Could you check a few things on this drawing? It's one solid part, dimensions in mm from its lowest x, y, z. Round coordinates to 2 decimals unless told otherwise and drop trailing zeros. Write each loop counter-clockwise with the first axis right and the second up, starting at its lowest first coordinate (ties: lowest second). Pieces come first, ordered by that corner, then holes. Notation, with made-up numbers: (23.5, 60) - (72.5, 60) arc R37 cw to (72.5, 96) - close; hole circle Ø3 at (-10.5, 49). An arc over 180 degrees is marked (long way). Use one line per item in the form item = value. Start each with the question number.
1. I want a section at A-A, the plane z = 3.5. State how many separate pieces and enclosed holes the cut face has, plus the area to 3 significant figures.
2. Will these pins go through, and if not, where does the flat tip stop? pin 1 (2.5 mm diameter, centred on y = 167, z = 2, fed in from -X); pin 2 (1 mm diameter, centred on x = 187.5, z = 4, fed in from +Y); pin 3 (1.5 mm diameter, centred on x = 130.5, z = 2.5, fed in from -Y).
3. I want a section at B-B, the plane x = 91. List the corners of the cut face in (y, z) for me.
4. I want a section at D-D, the plane x = 44. List the corners of the cut face in (y, z) for me.
5. If I drill on line 1 along Y through (x, z) = (92, 3.85); line 2 along X through (y, z) = (69, 3.7); line 3 along Y through (x, z) = (132.5, 2.9), over which ranges is the centre line in solid material (lowest first)?
6. I want a section at C-C, the plane y = 148. List the corners of the cut face in (x, z) for me, plus the area to 3 significant figures.
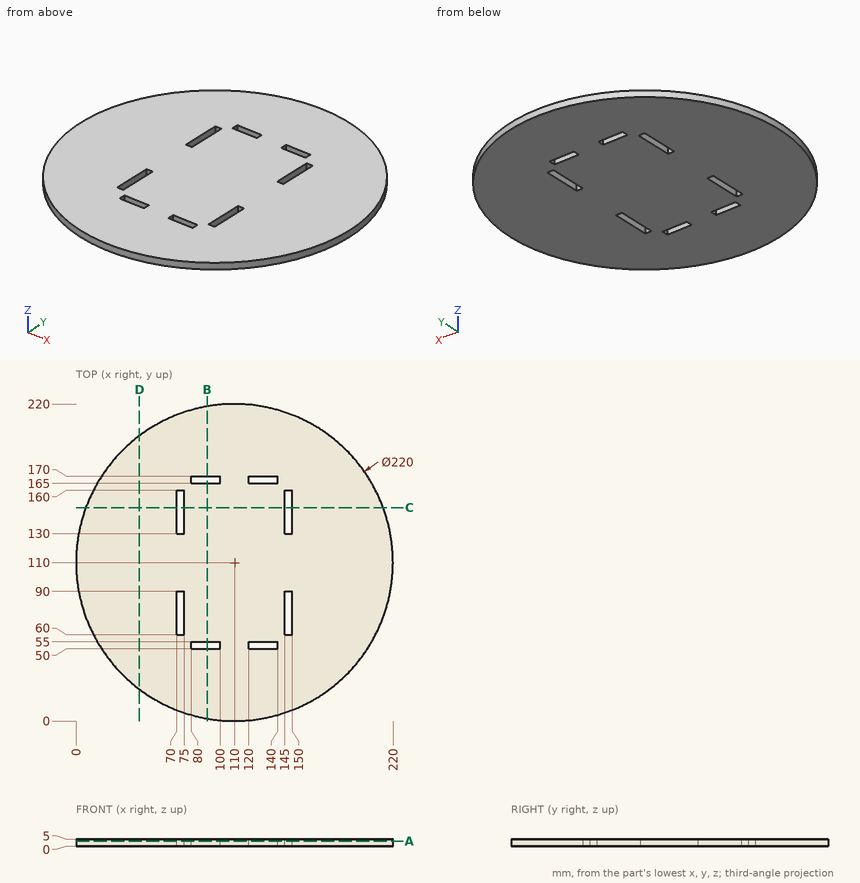
Model answer:
q1.separate_pieces = 1
q1.enclosed_holes = 8
q1.area = 37,000 mm2
q2.pin_1 = 15.17
q2.pin_2 = 188.56
q2.pin_3 = 1.79
q3.outline = (1.65, 0) - (50, 0) - (50, 5) - (1.65, 5) - close; (55, 0) - (165, 0) - (165, 5) - (55, 5) - close; (170, 0) - (218.35, 0) - (218.35, 5) - (170, 5) - close
q4.outline = (22, 0) - (198, 0) - (198, 5) - (22, 5) - close
q5.line_1 = 1.48 to 50, 55 to 165, 170 to 218.52
q5.line_2 = 7.93 to 70, 75 to 145, 150 to 212.07
q5.line_3 = 2.33 to 50, 55 to 165, 170 to 217.67
q6.outline = (6.77, 0) - (70, 0) - (70, 5) - (6.77, 5) - close; (75, 0) - (145, 0) - (145, 5) - (75, 5) - close; (150, 0) - (213.23, 0) - (213.23, 5) - (150, 5) - close
q6.area = 982 mm2
